Can you work these out from the drawing? Everything is in mm from the part's minimum corner. A direction names the side the tool comes from. Coordinates: 2 decimals unless noted, no trailing zeros. Order: outer loops, then holes, each group sorted by start corner. A loop starts at its lowest first (then second) coordinate and runs counter-clockwise, first axis right, second up. Notation, with made-up numbers: (55.25, 35.25) -> (68.25, 35.25) arc R34 ccw to (68.25, 71.25) -> close; hole circle Ø6 at (-14, -13.75). An arc over 180 degrees is marked (long way). Put each result on its own line as item: value. Start each with the question number.
Q1. If we section it at A-A (x = 73.5): Please give me the cut outline in (y, z) (1 decimal).
Q2. If we section it at C-C (z = 6.5): Please give me the cut outline in (x, y) (1 decimal).
Q3. Will these pins go through, and if not, where does the flat tip stop? pin 1 (3 mm diameter, centred on y = 10.5, z = 3.5, fed in from -X); pin 2 (1 mm diameter, centred on x = 69, y = 45.5, fed in from +Z).
Q4. If we section it at D-D (y = 52): Please give me the cut outline in (x, z), and give its area (3 significant figures).
Q5. For the marked faces 1 and 2, which set-ups out of +Z, -Z, +X, -X, +Y, -Y let a thin tool reach every point of the face, with its end or its side?
Q6. If we section it at B-B (y = 6): Please give me the cut outline in (x, z), and give its area (3 significant figures).
Q7. Please list where these lines run through material, in increasing order: line 1 along X through (y, z) = (30.5, 0.5); line 2 along X through (y, z) = (38.5, 1.5) (1 decimal); line 3 along Z through (x, y) = (75.5, 53).
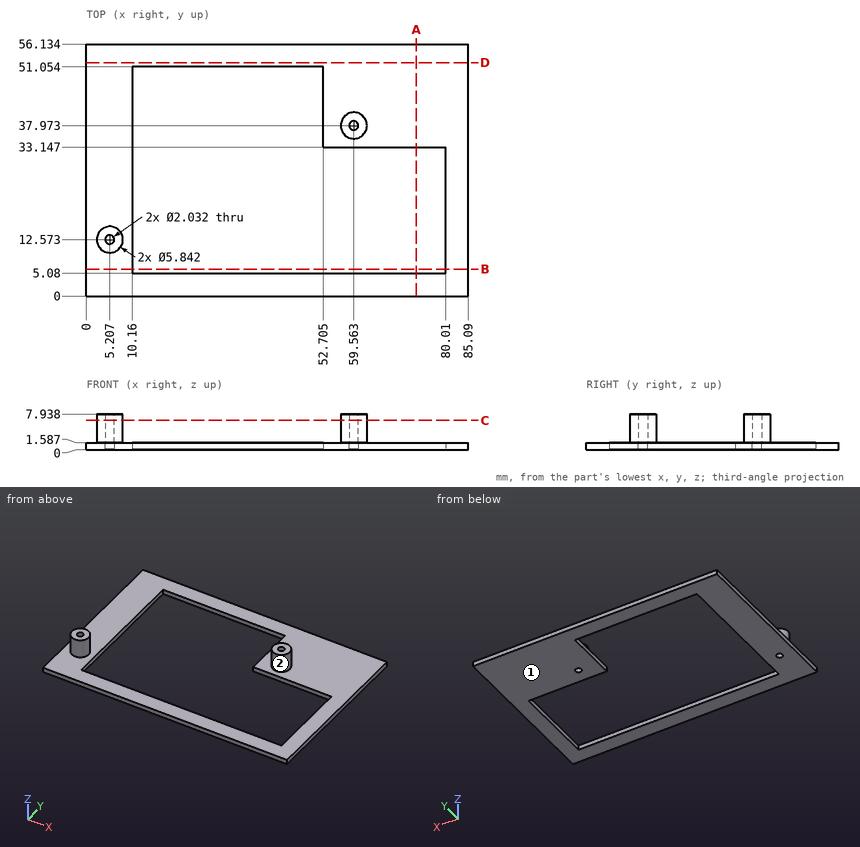
The answers:
1. outline: (0, 0) -> (5.1, 0) -> (5.1, 1.6) -> (0, 1.6) -> close; (33.1, 0) -> (56.1, 0) -> (56.1, 1.6) -> (33.1, 1.6) -> close
2. outline: circle Ø5.8 at (5.2, 12.6); circle Ø5.8 at (59.6, 38); hole circle Ø2 at (5.2, 12.6); hole circle Ø2 at (59.6, 38)
3. pin 1: x = 2.34
3. pin 2: z = 1.59
4. outline: (0, 0) -> (85.09, 0) -> (85.09, 1.59) -> (0, 1.59) -> close
4. area: 135 mm^2
5. face 1: -Z, +X, -X, +Y, -Y
5. face 2: +Z
6. outline: (0, 0) -> (10.16, 0) -> (10.16, 1.59) -> (0, 1.59) -> close; (80.01, 0) -> (85.09, 0) -> (85.09, 1.59) -> (80.01, 1.59) -> close
6. area: 24.2 mm^2
7. line 1: 0 to 10.16, 80.01 to 85.09
7. line 2: 0 to 10.2, 52.7 to 58.7, 60.4 to 85.1
7. line 3: 0 to 1.59
